Job drawing, mm, ordinate dimensions from the low corner. One solid piece. A direction names the side the tool comes from. Round coordinates to 2 decimals unless told otherwise and drop trailing zeros. Loops run counter-clockwise (first coordinate to the right, second up) from the corner with the lowest first, then second, coordinate; pieces in that order, holes last.
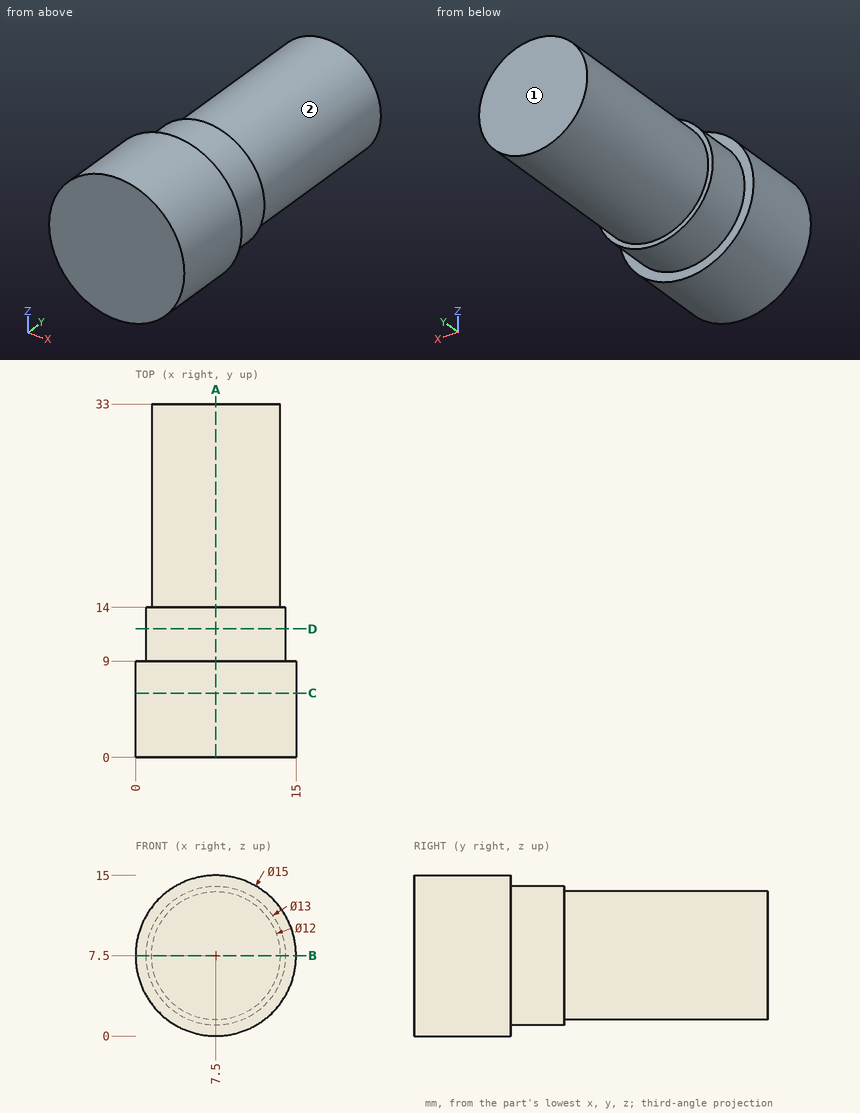
Item 1: Cut at C-C, the plane y = 6. Give the cut face in (x, z), plus the area to 3 significant figures.
Answers follow:
outline: circle Ø15 at (7.5, 7.5)
area: 177 mm2
Item 2: Cut at D-D, the plane y = 12. Give the cut face in (x, z), plus the area to 3 significant figures.
Answers follow:
outline: circle Ø13 at (7.5, 7.5)
area: 133 mm2
Item 3: Flat gauge pins, fed straight in: P1, Ø1.5, axis at y = 20, z = 3, coming from the +X side; P2, Ø8, axis at y = 22.5, z = 9.5, coming from the +X side; P3, Ø2, axis at x = 8, y = 18.5, coming from the -Z side. Where does each tip first touch, or does it go through?
Answers follow:
P1: stops at x = 12.18
P2: stops at x = 13.5
P3: stops at z = 1.5
Item 4: Probe line 1 (Y direction, x = 1.75, z = 5); line 2 (Y direction, x = 6.75, z = 14); line 3 (X direction, y = 2.5, z = 8.75). List the from-to ranges inside material, lowest first.
Answers follow:
line 1: y = 0 to 14
line 2: y = 0 to 9
line 3: x = 0.1 to 14.9
Item 5: Cut at A-A, the plane x = 7.5. Give the cut face in (y, z), plus the area to 3 significant figures.
Answers follow:
outline: (0, 0) - (9, 0) - (9, 1) - (14, 1) - (14, 1.5) - (33, 1.5) - (33, 13.5) - (14, 13.5) - (14, 14) - (9, 14) - (9, 15) - (0, 15) - close
area: 428 mm2
Item 6: Cut at B-B, the plane z = 7.5. Give the cut face in (x, y).
Answers follow:
outline: (0, 0) - (15, 0) - (15, 9) - (14, 9) - (14, 14) - (13.5, 14) - (13.5, 33) - (1.5, 33) - (1.5, 14) - (1, 14) - (1, 9) - (0, 9) - close
Item 7: 3-axis set-ups, long thin cutter, end or side, ignore diameter. For the marked faces 1 and 2: which of +Z, -Z, +X, -X, +Y, -Y reach the whole face in a straight line?
Answers follow:
face 1: +Z, -Z, +X, -X, +Y
face 2: +Y
